Here's how the part is built. I have some questions about the finished solid (model axes, mm). A direction names the side the tool comes from. Round coordinates to 2 decimals unless told otherwise and drop trailing zeros. Loops run counter-clockwise (first coordinate to the right, second up) from the corner with the lowest first, then second, coordinate; pieces in that order, holes last. Notation, with made-up numbers: (-0.75, -40) -> (49.25, -40) arc R26 cw to (49.25, -1) -> close; hole circle Ø9 at (6, 66). An arc over 180 degrees is marked (long way). Use CSV: the item, a comma, the result in double quotes. Start each with the question number.
from build123d import *

# Parameters (mm, degrees)
F1_DEPTH = 4


with BuildPart() as f1:
    # F0 (on Front) → F1 (new body)
    with BuildSketch(Plane.XZ):
        with BuildLine():
            Line((-19.608427, 12.045941), (-39.61654, 12.045941))
            Line((-39.61654, 12.045941), (-37.717187, -1.468657))
            ThreePointArc((-37.717187, -1.468657), (-36.376363, -3.938148), (-39.008427, -2.954059))
            Line((-39.008427, -2.954059), (-59.508427, -2.954059))
            Line((-59.508427, -2.954059), (-59.508427, -25.954059))
            Line((-59.508427, -25.954059), (-53.008427, -25.954059))
            Line((-53.008427, -25.954059), (-38.989615, -14.190879))
            ThreePointArc((-38.989615, -14.190879), (-37.508427, -12.454059), (-36.02724, -14.190879))
            Line((-36.02724, -14.190879), (-22.008427, -25.954059))
            Line((-22.008427, -25.954059), (-8.308427, -25.954059))
            Line((-8.308427, -25.954059), (-0.842829, -14.814868))
            ThreePointArc((-0.842829, -14.814868), (0.378701, -12.454237), (1.622211, -14.803363))
            Line((1.622211, -14.803363), (9.191573, -25.954059))
            Line((9.191573, -25.954059), (20.391573, -25.954059))
            Line((20.391573, -25.954059), (17.974175, -2.954059))
            Line((17.974175, -2.954059), (-3.108427, -2.954059))
            ThreePointArc((-3.108427, -2.954059), (-5.182452, -4.339879), (-5.669087, -1.893399))
            Line((-5.669087, -1.893399), (-19.608427, 12.045941))
        make_face()
    extrude(amount=F1_DEPTH)


solid = f1.part
Q1. I want a section at D-D, the plane z = 3.5. List the corners of the cut face in (x, y) for me, then the cut area to 3 significant figures.
Q2. I want a section at C-C, the plane x = -54. List the corners of the cut face in (y, z) for me.
Q3. I want a section at B-B, the plane z = -17.5. List the corners of the cut face in (x, y) for me, then the cut area to 3 significant figures.
Q4. If we mould it in two halves opening along Z, with no side actions, what happens to faces 6 (the cylindrical face through (0.333, -1.972, -12.455)), 7 (the flat face through (-20, 0, -11)), 8 (the flat face through (5.354, -1.972, -20.301))? For each: pulls with the +Z half, pulls with the -Z half, needs draft (parallel to the pull), parting line crosses it, or undercut.
Q5. I want a section at A-A, the plane y = -1.05. List the corners of the cut face in (x, z) for me, then the cut area to 3 significant figures.
Q6. Will these pins go through, and if not, where does the flat tip stop? pin 1 Ø1 at (x, y) = (-47, -1.5) entering from +Z; pin 2 Ø5 at (x, z) = (0.39, -13.95) entering from -Y; pin 3 Ø2.5 at (x, z) = (-37.51, -2.95) entering from +Y; pin 4 Ø1 at (y, z) = (-1, 8) entering from -X.
Q7. I need wall thicknesses on line 1 along X through (y, z) = (-1.95, -21); line 2 along X through (y, z) = (-1.55, -17.5); line 3 along Z through (x, y) = (-37.5, -1.2). Which ranges of each line are inside material? Lowest first, please.
Q8. For faces 1 (the flat face through (-4.628, -1.972, -20.462)), 2 (the flat face through (-59.508, -2, -14)), 3 (the flat face through (8, -2, -2.954)), 4 (the flat face through (-56, -2, -25.954)), 5 (the flat face through (-38.68, -1.97, 5.38)), which set-ups out of +Z, -Z, +X, -X, +Y, -Y let a thin tool reach every point of the face, with its end or its side?
Values found:
1,outline,"(-38.42, -4) -> (-11.06, -4) -> (-11.06, 0) -> (-38.42, 0) -> close"
1,area,"109 mm2"
2,outline,"(-4, -25.95) -> (0, -25.95) -> (0, -2.95) -> (-4, -2.95) -> close"
3,outline,"(-59.51, -4) -> (-42.93, -4) -> (-42.93, 0) -> (-59.51, 0) -> close; (-32.08, -4) -> (-2.64, -4) -> (-2.64, 0) -> (-32.08, 0) -> close; (3.45, -4) -> (19.5, -4) -> (19.5, 0) -> (3.45, 0) -> close"
3,area,"248 mm2"
4,face 6,"undercut"
4,face 7,"needs draft"
4,face 8,"pulls with the -Z half"
5,outline,"(-59.51, -25.95) -> (-53.01, -25.95) -> (-38.99, -14.19) arc R1.5 cw (long way) to (-36.03, -14.19) -> (-22.01, -25.95) -> (-8.31, -25.95) -> (-0.84, -14.81) arc R1.5 cw (long way) to (1.62, -14.8) -> (9.19, -25.95) -> (20.39, -25.95) -> (17.97, -2.95) -> (-3.11, -2.95) arc R1.5 cw (long way) to (-5.67, -1.89) -> (-19.61, 12.05) -> (-39.62, 12.05) -> (-37.72, -1.47) arc R1.5 cw (long way) to (-39.01, -2.95) -> (-59.51, -2.95) -> close"
5,area,"1,880 mm2"
6,pin 1,"z = -2.95"
6,pin 2,"y = -4"
6,pin 3,"through"
6,pin 4,"x = -39.12"
7,line 1,"-59.51 to -47.1, -27.91 to -4.99, 5.83 to 19.87"
7,line 2,"-59.51 to -42.93, -32.08 to -2.64, 3.45 to 19.5"
7,line 3,"-12.45 to -4.45, -1.45 to 12.05"
8,face 1,"-Z, +Y, -Y"
8,face 2,"+Z, -Z, -X, +Y, -Y"
8,face 3,"+Z, +X, +Y, -Y"
8,face 4,"-Z, +X, -X, +Y, -Y"
8,face 5,"-X, +Y, -Y"
